Here's how the part is built. I have some questions about the finished solid (model axes, mm). A direction names the side the tool comes from. Coordinates: 2 decimals unless noted, no trailing zeros. Put each result on its own line as item: value. Start each with the question number.
Item 1: If we mould it in two halves opening along Y, with no side actions, what happens to faces 1 (the face through (-0.14, 0.13, 13.52)), 2 (the face through (2.88, -1.57, 37.57)), 3 (the face through (1.5, -1.4, 0)), 4 (the face through (-0.382, -1.574, 69.761))? For each: released by +Y, released by -Y, zero draft, split by the parting line, or undercut.
Item 2: I need wall thicknesses on line 1 (Y direction, x = 0.75, z = 65.5); line 2 (Y direction, x = 1.5, z = 68); line 3 (X direction, y = 2, z = 3). Which ranges of each line are inside material? Lowest first, please. Write a range as [from, to].
Item 3: For pin 1 (1 mm diameter, centred on x = 2.5, y = -1, fed in from -Z); pin 2 (3 mm diameter, centred on x = 0.11, y = 0, fed in from -Z); pin 3 (3 mm diameter, centred on x = 0.11, y = 0, fed in from +Z), each with a flat end and sliding along its axis, tell me the tip position at first contact or that it passes through.
Item 4: On a 3-axis mill with a long thin cutter (end or side, diameter ignored), from which of +Z, -Z, +X, -X, +Y, -Y can I reach the whole of each face in a straight line? I mean faces 5 (the face through (0, 3.175, 38)), 6 (the face through (1.725, -0.358, 6.439)). Say none if no direction works.
Autodesk Inventor part; units mm, degrees
ref_plane "Work Plane1" through (-1.711, 0.0003, 0) normal (0, 1, 0) x (1, 0, 0)
ref_plane "YZ Plane" through (0, 0, 0) normal (1, 0, 0) x (0, 1, 0)
ref_plane "XZ Plane" through (0, 0, 0) normal (0, 1, 0) x (-1, 0, 0)
sketch "Sketch1" plane through (0, 0, 0) normal (0, 0, 1) x (1, 0, 0)
  line L0 (1.9552, -3.1747) -> (-1.711, -3.1747)
  line L1 (-1.711, -3.1747) -> (-3.5441, 0.0003)
  line L2 (-3.5441, 0.0003) -> (-1.711, 3.1753)
  line L3 (-1.711, 3.1753) -> (1.9552, 3.1753)
  line L4 (1.9552, 3.1753) -> (3.7883, 0.0003)
  line L5 (3.7883, 0.0003) -> (1.9552, -3.1747)
  point P0 (0.1221, 0.0003)
  dimension "d0" = 6.35
extrude "Extrusion1" add sketch "Sketch1" along normal blind 76.2
ref_plane "Work Plane1" through (-1.711, 0.0003, 0) normal (0, 1, 0) x (1, 0, 0)
sketch "Sketch3" plane through (-1.711, 0.0003, 0) normal (0, 1, 0) x (1, 0, 0)
  line L0 (-1.3251, 0) -> (4.9741, 0)
  line L1 (5.4821, -0.508) -> (5.4821, -75.692)
  line L2 (4.9741, -76.2) -> (-1.3251, -76.2)
  line L3 (-1.8331, -75.692) -> (-1.8331, -0.508)
  line L4 (-1.8331, -0.508) -> (-1.3251, 0)
  line L5 (4.9741, 0) -> (5.4821, -0.508)
  line L6 (-1.3251, -76.2) -> (-1.8331, -75.692)
  line L7 (5.4821, -75.692) -> (4.9741, -76.2)
  line L8 (-1.8331, 0) -> (-1.8331, -76.2)
  line L9 (3.6662, 0) -> (5.4993, 0)
  line L10 (1.8245, 0) -> (1.8245, -76.2)
  point P0 (-1.8331, 0)
  point P1 (5.4821, -76.2)
  point P2 (5.4821, 0)
  point P3 (-1.8331, -76.2)
  dimension "d5" = 0.508
  dimension "d6" = 0.508
  dimension "d7" = 0.508
  dimension "d8" = 0.508
  dimension "d9" = 0.508
  dimension "d10" = 0.508
  dimension "d11" = 0.508
  dimension "d12" = 0.508
  dimension "d13" = 7.3152
  dimension "d14" = 0
  dimension "d15" = 76.2
  dimension "d16" = 0
revolve "Revolution1" cut sketch "Sketch3" angle 360 about axis through (0.1135, 0.0003, 0) along (0, 0, 1) keep common part contours L0 L5 L1 L7 L2 L10
sketch "Sketch5" plane through (0.1135, 0.0003, 76.2) normal (0, 0, 1) x (1, 0, 0)
  circle A0 centre (0, 0) radius 3.1496
hole "Hole2" at (0.1135, 0.0003, 76.2) at (0.1135, 0.0003, 76.2) direction (0, 0, -1) diameter 3.302 depth 12.7 tip angle 118
sketch "Sketch6" plane through (0.1135, 0.0003, 0) normal (0, 0, -1) x (-1, 0, 0)
  circle A0 centre (0, 0) radius 3.1496
hole "Hole3" at (0.1135, 0.0003, 0) direction (0, 0, 1) diameter 3.302 depth 12.7 tip angle 118
properties part number "275-1020" material "Steel"
Calculated:
1. face 1: undercut
1. face 2: released by -Y
1. face 3: zero draft
1. face 4: undercut
2. line 1: y = [-3.17, -1.52], [1.52, 3.18]
2. line 2: y = [-3.17, -0.9], [0.9, 3.18]
2. line 3: x = [-2.39, 2.63]
3. pin 1: stops at z = 0
3. pin 2: stops at z = 12.79
3. pin 3: stops at z = 63.41
4. face 5: +Z, -Z, +X, -X, +Y
4. face 6: -Z
